For this review, use the dimensioned drawing (mm, ordinates from the lowest corner) and the shaded views. A direction names the side the tool comes from. Round coordinates to 2 decimals unless told otherwise and drop trailing zeros. Order: outer loops, then holes, each group sorted by start corner. A loop starts at its lowest first (then second) coordinate and runs counter-clockwise, first axis right, second up. Notation, with made-up numbers: M 69,65 L 85,65 A9 ccw 85,80 Z; hole C 59,-30 d7. An arc over 180 degrees is marked long. Put each result on its own line as item: value.
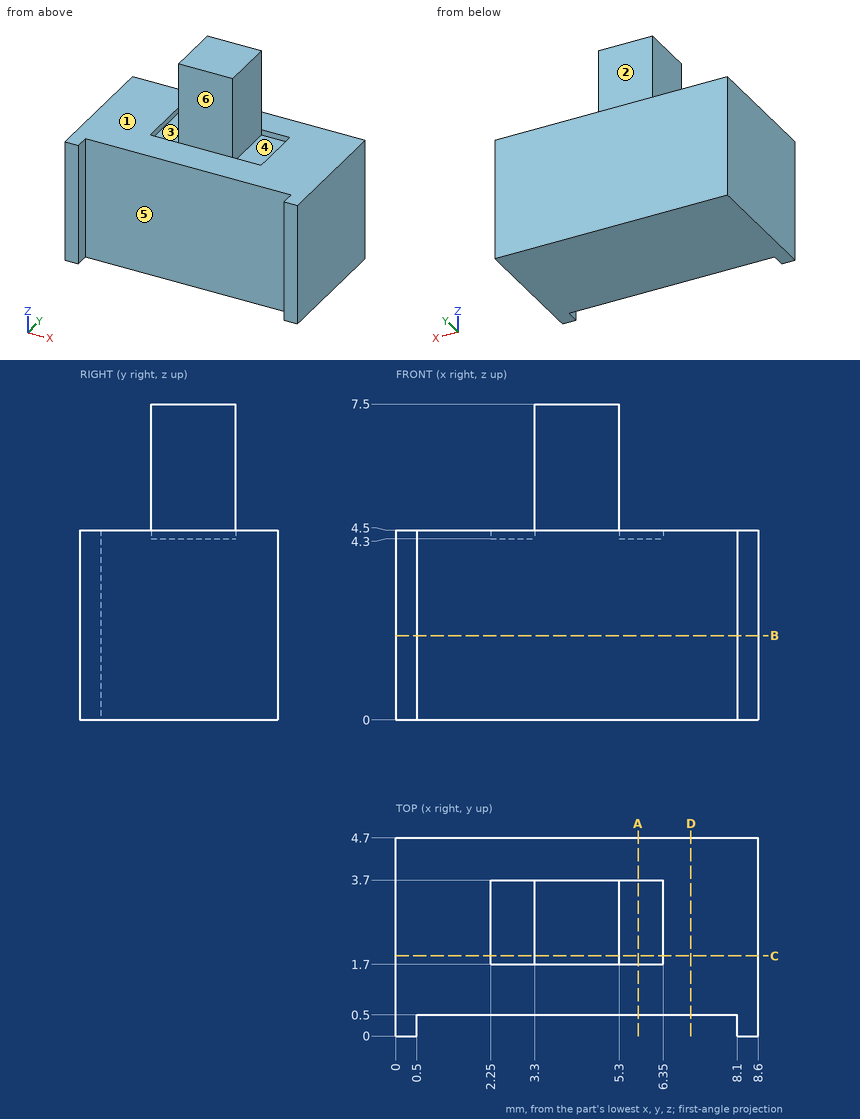
(1) To check wall thickness, follow L1, parallel to Z at x = 6, y = 3.65; L2, parallel to Y at x = 4.75, z = 1.75; L3, parallel to Y at x = 4.5, z = 6. State the ranges of each line that lie inside material, in increasing order.
A:
L1: z = 0 to 4.3
L2: y = 0.5 to 4.7
L3: y = 1.7 to 3.7
(2) Add section D-D on x = 7. Give the boundary of the cut face in (y, z).
A:
outline: M 0.5,0 L 4.7,0 L 4.7,4.5 L 0.5,4.5 Z
(3) Draft analysis for pull direction Y (two halves, no side actions). For the marked faces 1, 2 and 3, state which applies: released by +Y, released by -Y, zero draft, split by the parting line, or undercut.
A:
face 1: zero draft
face 2: released by +Y
face 3: undercut
(4) Add section B-B on z = 2. Give the boundary of the cut face in (x, y), then the cut area to 3 significant figures.
A:
outline: M 0,0 L 0.5,0 L 0.5,0.5 L 8.1,0.5 L 8.1,0 L 8.6,0 L 8.6,4.7 L 0,4.7 Z
area: 36.6 mm2
(5) Add section C-C on y = 1.9. Give the boundary of the cut face in (x, z), then the cut area to 3 significant figures.
A:
outline: M 0,0 L 8.6,0 L 8.6,4.5 L 6.35,4.5 L 6.35,4.3 L 5.3,4.3 L 5.3,7.5 L 3.3,7.5 L 3.3,4.3 L 2.25,4.3 L 2.25,4.5 L 0,4.5 Z
area: 44.3 mm2
(6) For the marked faces 4, 5 and 6, list the 3-axis set-ups (+Z, -Z, +X, -X, +Y, -Y) from which the entire face can be reached by the end or side of a thin tool; tool diameter is ignored.
A:
face 4: +Z
face 5: +Z, -Z, -Y
face 6: +Z, +X, -X, -Y
(7) Insertion check: pin 1 Ø1.3 at (x, z) = (3, 1) entering from -Y; pin 2 Ø1.6 at (x, z) = (5, 5.5) entering from +Y; pin 3 Ø1 at (x, z) = (4, 6.5) entering from -Y. Each pin has a flat end and moves straight along its axis. Give the tip position at first contact, or say it passes through.
A:
pin 1: stops at y = 0.5
pin 2: stops at y = 3.7
pin 3: stops at y = 1.7
(8) Add section A-A on x = 5.75. Give the boundary of the cut face in (y, z), then the cut area to 3 significant figures.
A:
outline: M 0.5,0 L 4.7,0 L 4.7,4.5 L 3.7,4.5 L 3.7,4.3 L 1.7,4.3 L 1.7,4.5 L 0.5,4.5 Z
area: 18.5 mm2
